```python
from build123d import *

# Parameters (mm, degrees)
SKETCH1_R           = 3.4925
SKETCH1_R_2         = 0.8509
BOSS_EXTRUDE1_DEPTH = 15.875
SKETCH2_R           = 3.4925
BOSS_EXTRUDE2_DEPTH = 2.54
SKETCH3_R           = 6.0325
BOSS_EXTRUDE3_DEPTH = 6.35
SKETCH4_R           = 0.889
CUT_EXTRUDE1_DEPTH  = 3.5


with BuildPart() as part:
    # Sketch1 → Boss-Extrude1 (new body)
    with BuildSketch(Plane.XY):
        Circle(SKETCH1_R)
        Circle(SKETCH1_R_2, mode=Mode.SUBTRACT)
    extrude(amount=BOSS_EXTRUDE1_DEPTH)

    # Sketch2 → Boss-Extrude2 (add)
    with BuildSketch(Plane.XY.offset(15.875)):
        Circle(SKETCH2_R)
    extrude(amount=BOSS_EXTRUDE2_DEPTH)

    # Sketch3 → Boss-Extrude3 (add)
    with BuildSketch(Plane.XY.offset(18.415)):
        Circle(SKETCH3_R)
    extrude(amount=BOSS_EXTRUDE3_DEPTH)

    # Sketch4 → Cut-Extrude1 (cut)
    with BuildSketch(Plane.ZY.offset(3.4925)):
        with Locations((2.54, 0)):
            Circle(SKETCH4_R)
        with Locations((8.89, 0)):
            Circle(SKETCH4_R)
    extrude(amount=-CUT_EXTRUDE1_DEPTH, mode=Mode.SUBTRACT)


solid = part.part
```
The model under review builds one solid part; all positions refer to its coordinate system, in mm. A direction names the side the tool comes from. Round coordinates to 2 decimals unless told otherwise and drop trailing zeros. Loops run counter-clockwise (first coordinate to the right, second up) from the corner with the lowest first, then second, coordinate; pieces in that order, holes last. Notation, with made-up numbers: (-31.75, 61.25) -> (-2.75, 61.25) arc R15 cw to (-2.75, 72.25) -> close; hole circle Ø5 at (-23, 12.5). An arc over 180 degrees is marked (long way). Answer as a JSON object with one key per item and string values. Group by question number.
1) We need section A-A on y = 0. Write out the cut boundary in (x, z) (1 decimal), then the cut area to 3 significant figures.
2) We need section B-B on x = -3. Write out the cut boundary in (y, z) (3 decimals), then the cut area to 3 significant figures.
3) For pin 1 Ø4 at (x, z) = (-2, 13) entering from -Y; pin 2 Ø3 at (y, z) = (0, 8.89) entering from +X; pin 3 Ø3 at (y, z) = (0, 2.54) entering from -X, all flat-tipped, find the tip position at first contact; note any pin that passes through.
4) For faces 4 (the face through (-2.156, 0.267, 9.738)), 5 (the face through (0, 0, 15.875)), 6 (the face through (5.754, 1.812, 21.546)), list the 3-axis set-ups (+Z, -Z, +X, -X, +Y, -Y) from which the entire face can be reached by the end or side of a thin tool; tool diameter is ignored.
5) We need section D-D on x = 2.5. Write out the cut boundary in (y, z) (3 decimals), then the cut area to 3 significant figures.
6) For line 1 (X direction, y = 0, z = 10); line 2 (Z direction, x = 5, y = -1) (3 decimals), list the stretches that pass through material, from the lowest coordinate up. Write a range as [from, to].
7) Mouldability with a two-part tool opening along Y and no side actions: class faces 1 (the face through (0.81, 0.26, 7.83)), 2 (the face through (3, -3, 18.415)), 3 (the face through (3.33, 1.05, 9.08)) as released by +Y, released by -Y, zero draft, split by the parting line, or undercut.
8) We need section C-C on z = 3.75. Write out the cut boundary in (x, y) (1 decimal), then the cut area to 3 significant figures.
Result set:
{
 "1": {"outline": "(-6, 18.4) -> (-3.5, 18.4) -> (-3.5, 9.8) -> (-0.9, 9.8) -> (-0.9, 15.9) -> (0.9, 15.9) -> (0.9, 0) -> (3.5, 0) -> (3.5, 18.4) -> (6, 18.4) -> (6, 24.8) -> (-6, 24.8) -> close; (-3.5, 0) -> (-0.9, 0) -> (-0.9, 1.7) -> (-3.5, 1.7) -> close; (-3.5, 3.4) -> (-0.9, 3.4) -> (-0.9, 8) -> (-3.5, 8) -> close", "area": "169 mm²"},
 "2": {"outline": "(-5.234, 18.415) -> (-1.788, 18.415) -> (-1.788, 0) -> (1.788, 0) -> (1.788, 18.415) -> (5.234, 18.415) -> (5.234, 24.765) -> (-5.234, 24.765) -> close; hole circle Ø1.778 at (0, 2.54); hole circle Ø1.778 at (0, 8.89)", "area": "127 mm²"},
 "3": {"pin 1": "y = -3.49", "pin 2": "x = 3.49", "pin 3": "x = -3.49"},
 "4": {"face 4": "-X", "face 5": "-Z", "face 6": "+Z, -Z"},
 "5": {"outline": "(-5.49, 18.415) -> (-2.439, 18.415) -> (-2.439, 0) -> (2.439, 0) -> (2.439, 18.415) -> (5.49, 18.415) -> (5.49, 24.765) -> (-5.49, 24.765) -> close", "area": "160 mm²"},
 "6": {"line 1": "[-3.49, -0.85], [0.85, 3.49]", "line 2": "[18.415, 24.765]"},
 "7": {"face 1": "undercut", "face 2": "zero draft", "face 3": "split by the parting line"},
 "8": {"outline": "circle Ø7 at (0, 0); hole circle Ø1.7 at (0, 0)", "area": "36.0 mm²"}
}
